Read the model definition and answer for the solid it produces. Units are mm, in the model's axes. Coordinates: 2 decimals unless noted, no trailing zeros. Loops run counter-clockwise (first coordinate to the right, second up) from the corner with the lowest first, then second, coordinate; pieces in that order, holes last.
Q1. Flat-ended cylindrical pins translate along their axes: P1, Ø4, axis at y = 0.5, z = 108, coming from the -X side; P2, Ø1.9, axis at y = -4, z = 82.5, coming from the +X side; P3, Ø2, axis at y = -2.5, z = 226, coming from the -X side; P4, Ø1.5, axis at x = 2.5, y = 6.5, coming from the -Z side. Find the tip coordinate at first contact, or state that the pin passes through.
Q2. Section A-A (y = 0) is taken. Give the vertices of the cut face in (x, z).
Q3. Straight lines are drawn through the part: line 1 (X direction, y = 0, z = 158.5); line 2 (X direction, y = -8.25, z = 206.5). For each, find the intervals that lie inside material, in ascending order.
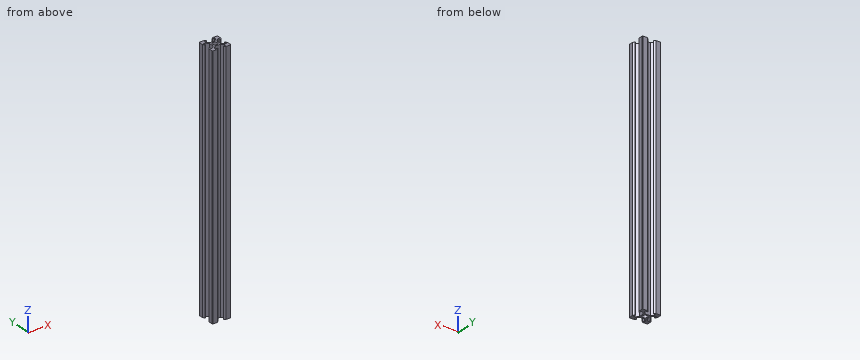
from build123d import *

# Parameters (mm, degrees)
CROQUIS1_R              = 2.5
SALIENTE_EXTRUIR1_DEPTH = 350
CUT_EXTRUDE1_DEPTH      = 47
CUT_EXTRUDE1_DEPTH_BACK = 40
SKETCH2_W               = 139.582587955
SKETCH2_H               = 242.432915921


with BuildPart() as part:
    # Croquis1 → Saliente-Extruir1 (new body)
    with BuildSketch(Plane.XY):
        with BuildLine():
            Line((-4.6, 10), (-3.1, 8.5))
            Line((-3.1, 8.5), (-3.1, 8.2))
            Line((-3.1, 8.2), (-5.5, 8.2))
            Line((-5.5, 8.2), (-5.5, 6.560660172))
            Line((-5.5, 6.560660172), (-2.84, 3.900660172))
            Line((-2.84, 3.900660172), (0, 3.900660172))
            Line((0, 3.900660172), (2.84, 3.900660172))
            Line((2.84, 3.900660172), (5.5, 6.560660172))
            Line((5.5, 6.560660172), (5.5, 8.2))
            Line((5.5, 8.2), (3.1, 8.2))
            Line((3.1, 8.2), (3.1, 8.5))
            Line((3.1, 8.5), (4.6, 10))
            Line((4.6, 10), (9.25, 10))
            ThreePointArc((9.25, 10), (9.780330086, 9.780330086), (10, 9.25))
            Line((10, 9.25), (10, 4.6))
            Line((10, 4.6), (8.5, 3.1))
            Line((8.5, 3.1), (8.2, 3.1))
            Line((8.2, 3.1), (8.2, 5.5))
            Line((8.2, 5.5), (6.560660172, 5.5))
            Line((6.560660172, 5.5), (3.900660172, 2.84))
            Line((3.900660172, 2.84), (3.900660172, 0))
            Line((3.900660172, 0), (3.900660172, -2.84))
            Line((3.900660172, -2.84), (6.560660172, -5.5))
            Line((6.560660172, -5.5), (8.2, -5.5))
            Line((8.2, -5.5), (8.2, -3.1))
            Line((8.2, -3.1), (8.5, -3.1))
            Line((8.5, -3.1), (10, -4.6))
            Line((10, -4.6), (10, -9.25))
            ThreePointArc((10, -9.25), (9.780330086, -9.780330086), (9.25, -10))
            Line((9.25, -10), (4.6, -10))
            Line((4.6, -10), (3.1, -8.5))
            Line((3.1, -8.5), (3.1, -8.2))
            Line((3.1, -8.2), (5.5, -8.2))
            Line((5.5, -8.2), (5.5, -6.560660172))
            Line((5.5, -6.560660172), (2.84, -3.900660172))
            Line((2.84, -3.900660172), (0, -3.900660172))
            Line((0, -3.900660172), (-2.84, -3.900660172))
            Line((-2.84, -3.900660172), (-5.5, -6.560660172))
            Line((-5.5, -6.560660172), (-5.5, -8.2))
            Line((-5.5, -8.2), (-3.1, -8.2))
            Line((-3.1, -8.2), (-3.1, -8.5))
            Line((-3.1, -8.5), (-4.6, -10))
            Line((-4.6, -10), (-9.25, -10))
            ThreePointArc((-9.25, -10), (-9.780330086, -9.780330086), (-10, -9.25))
            Line((-10, -9.25), (-10, -4.6))
            Line((-10, -4.6), (-8.5, -3.1))
            Line((-8.5, -3.1), (-8.2, -3.1))
            Line((-8.2, -3.1), (-8.2, -5.5))
            Line((-8.2, -5.5), (-6.560660172, -5.5))
            Line((-6.560660172, -5.5), (-3.900660172, -2.84))
            Line((-3.900660172, -2.84), (-3.900660172, 0))
            Line((-3.900660172, 0), (-3.900660172, 2.84))
            Line((-3.900660172, 2.84), (-6.560660172, 5.5))
            Line((-6.560660172, 5.5), (-8.2, 5.5))
            Line((-8.2, 5.5), (-8.2, 3.1))
            Line((-8.2, 3.1), (-8.5, 3.1))
            Line((-8.5, 3.1), (-10, 4.6))
            Line((-10, 4.6), (-10, 9.25))
            ThreePointArc((-10, 9.25), (-9.780330086, 9.780330086), (-9.25, 10))
            Line((-9.25, 10), (-4.6, 10))
        make_face()
        Circle(CROQUIS1_R, mode=Mode.SUBTRACT)
    extrude(amount=SALIENTE_EXTRUIR1_DEPTH)

    # Sketch2 → Cut-Extrude1 (cut, two sides: drawn at the far end of the back side and taken through both)
    with BuildSketch(Plane(origin=(0, 0, 0), x_dir=(1, 0, 0), z_dir=(0, 1, 0)).offset(-CUT_EXTRUDE1_DEPTH_BACK)):
        with Locations((12.355396541, -391.216457961)):
            Rectangle(SKETCH2_W, SKETCH2_H)
    extrude(amount=CUT_EXTRUDE1_DEPTH + CUT_EXTRUDE1_DEPTH_BACK, mode=Mode.SUBTRACT)


solid = part.part
Numbers:
1. P1: stops at x = -3.9
1. P2: stops at x = 10
1. P3: stops at x = -8.9
1. P4: passes through
2. outline: (-3.9, 0) - (-2.5, 0) - (-2.5, 270) - (-3.9, 270) - close; (2.5, 0) - (3.9, 0) - (3.9, 270) - (2.5, 270) - close
3. line 1: x = -3.9 to -2.5, 2.5 to 3.9
3. line 2: x = -10 to -3.1, 3.1 to 10
